Read the model definition and answer for the solid it produces. Units are mm, in the model's axes. A direction names the side the tool comes from. Round coordinates to 2 decimals unless told otherwise and drop trailing zeros. Write each loop counter-clockwise with the first axis right and the second up, starting at its lowest first coordinate (ties: lowest second). Pieces come first, ordered by that corner, then holes. Notation, with made-up numbers: (15.5, 85) -> (40.5, 85) arc R4 ccw to (40.5, 89) -> close; hole circle Ø4 at (-9, -17). An arc over 180 degrees is marked (long way). Return JSON: item names as keys, results as strings. Group by question number.
(1) For faces 1 (the flat face through (62, 2, 28.829)), 2 (the flat face through (-38, 2, 47.625)), 3 (the flat face through (-62, 2, -47.371)), 4 (the flat face through (-62, 2, -15.875)), determine the directions among +Z, -Z, +X, -X, +Y, -Y from which every point of the face is accessible in a straight line to the end or side of a thin tool.
(2) A cutting plane is placed at A-A on x = 2. Give the vertices of the cut face in (y, z) (3 decimals), then the cut area to 3 significant figures.
(3) Straight lines are drawn through the part: line 1 (X direction, y = 1.8, z = 14); line 2 (Z direction, x = 36.5, y = 2.15) (3 decimals). For each, find the intervals that lie inside material, in ascending order.
(4) The mould has two halves that part along Z. Classify faces 5 (the flat face through (0, 2, 47.625)), 6 (the flat face through (-62, 2, -34.671)), 7 (the flat face through (-60.198, 2, 25)), 8 (the flat face through (9.334, 2, 51)): released by +Z, released by -Z, zero draft, split by the parting line, or undercut.
(5) Given pin 1 (1.6 mm diameter, centred on x = -61.5, y = 1.5, fed in from +Z) (3 decimals); pin 2 (1 mm diameter, centred on y = 2, z = 26, fed in from +X); pin 3 (1 mm diameter, centred on y = 1.5, z = 49.5, fed in from -X), each flat-ended and moving along its own axis, determine where each tip first touches the part or whether it passes through.
```python
from build123d import *

# Parameters (mm, degrees)
SKETCH1_W           = 127
SKETCH1_H           = 107.95
BOSS_EXTRUDE1_DEPTH = 3.175
SKETCH2_W           = 3.302
SKETCH2_H           = 6.604
CUT_EXTRUDE1_DEPTH  = 84.400427157


with BuildPart() as part:
    # Sketch1 → Boss-Extrude1 (new body)
    with BuildSketch(Plane(origin=(0, 0, 0), x_dir=(1, 0, 0), z_dir=(0, 1, 0))):
        Rectangle(SKETCH1_W, SKETCH1_H)
    extrude(amount=BOSS_EXTRUDE1_DEPTH)

    # Sketch2 → Cut-Extrude1 (cut, through all)
    with BuildSketch(Plane.XZ):
        Polygon((-34.7345, 47.625), (-41.4655, 47.625), (-41.4655, 54.229), (-47.4345, 54.229), (-47.4345, 47.625), (-60.198, 47.625), (-63.5, 47.625), (-63.5, 54.229), (-63.5, 63.03162391), (63.5, 63.03162391), (63.5, 54.229), (63.5, 47.625), (60.198, 47.625), (47.4345, 47.625), (47.4345, 54.229), (41.4655, 54.229), (41.4655, 47.625), (34.7345, 47.625), (34.7345, 54.229), (28.7655, 54.229), (28.7655, 47.625), (22.0345, 47.625), (22.0345, 54.229), (16.0655, 54.229), (16.0655, 47.625), (9.3345, 47.625), (9.3345, 54.229), (3.3655, 54.229), (3.3655, 47.625), (-3.3655, 47.625), (-3.3655, 54.229), (-9.3345, 54.229), (-9.3345, 47.625), (-16.0655, 47.625), (-16.0655, 54.229), (-22.0345, 54.229), (-22.0345, 47.625), (-28.7655, 47.625), (-28.7655, 54.229), (-34.7345, 54.229), align=None)
        with Locations((61.849, 38.227)):
            Rectangle(SKETCH2_W, SKETCH2_H)
        with Locations((61.849, 25.527)):
            Rectangle(SKETCH2_W, SKETCH2_H)
        with Locations((61.849, 12.827)):
            Rectangle(SKETCH2_W, SKETCH2_H)
        with Locations((61.849, 0.127)):
            Rectangle(SKETCH2_W, SKETCH2_H)
        with Locations((61.849, -12.573)):
            Rectangle(SKETCH2_W, SKETCH2_H)
        with Locations((61.849, -25.273)):
            Rectangle(SKETCH2_W, SKETCH2_H)
        with Locations((61.849, -37.973)):
            Rectangle(SKETCH2_W, SKETCH2_H)
        with Locations((-61.849, -37.973)):
            Rectangle(SKETCH2_W, SKETCH2_H)
        with Locations((-61.849, -25.273)):
            Rectangle(SKETCH2_W, SKETCH2_H)
        with Locations((-61.849, -12.573)):
            Rectangle(SKETCH2_W, SKETCH2_H)
        with Locations((-61.849, 0.127)):
            Rectangle(SKETCH2_W, SKETCH2_H)
        with Locations((-61.849, 12.827)):
            Rectangle(SKETCH2_W, SKETCH2_H)
        with Locations((-61.849, 25.527)):
            Rectangle(SKETCH2_W, SKETCH2_H)
        with Locations((-61.849, 38.227)):
            Rectangle(SKETCH2_W, SKETCH2_H)
        with Locations((61.849, -50.673)):
            Rectangle(SKETCH2_W, SKETCH2_H)
        with Locations((-61.849, -50.673)):
            Rectangle(SKETCH2_W, SKETCH2_H)
    extrude(amount=-CUT_EXTRUDE1_DEPTH, mode=Mode.SUBTRACT)


solid = part.part
```
Checks:
{
 "1": {"face 1": "+X, +Y, -Y", "face 2": "+Z, +Y, -Y", "face 3": "-Z, -X, +Y, -Y", "face 4": "-X, +Y, -Y"},
 "2": {"outline": "(0, -53.975) -> (3.175, -53.975) -> (3.175, 47.625) -> (0, 47.625) -> close", "area": "323 mm^2"},
 "3": {"line 1": "x = -60.2 to 60.2", "line 2": "z = -53.975 to 47.625"},
 "4": {"face 5": "released by +Z", "face 6": "undercut", "face 7": "undercut", "face 8": "zero draft"},
 "5": {"pin 1": "stops at z = 47.625", "pin 2": "stops at x = 60.2", "pin 3": "stops at x = -47.43"}
}
